Can you work these out from the model? Positions are in its coordinate system, mm. Face numbers are marked on the shaded views. Round coordinates to 2 decimals unless told otherwise and drop trailing zeros. Write each loop counter-clockwise with the first axis right and the second up, starting at its lowest first coordinate (ties: lowest second). Pieces come first, ordered by that corner, then holes. Notation, with made-up numbers: M 38.5,17.5 L 49.5,17.5 A27 ccw 49.5,48.5 Z; hole C 1.5,86.5 d1. An arc over 180 degrees is marked long. Answer in a Markdown table with one row per item. Add a question column.
(1) If we mould it in two halves opening along Z, with no side actions, what happens to the marked faces 1, 2 and 3? For each: released by +Z, released by -Z, zero draft, split by the parting line, or undercut.
(2) I'm going to push flat-ended pins straight in: pin 1 (4 mm diameter, centred on x = 23, y = 44.5, fed in from +Z); pin 2 (8 mm diameter, centred on y = 57.5, z = -13.5, fed in from +X); pin 3 (2.5 mm diameter, centred on x = 9.29, y = 58, fed in from -Z); pin 4 (4 mm diameter, centred on x = 23.5, y = 39, fed in from -Z). Where does each tip first touch, or does it pass through?
(3) Suppose I cut it at C-C, the plane x = 11.75. Write out the boundary of the cut face in (y, z), then the cut area to 3 significant figures.
(4) Suppose I cut it at A-A, the plane y = 64. Write out the boundary of the cut face in (x, z).
(5) Suppose I cut it at D-D, the plane z = -16.5. Write out the boundary of the cut face in (x, y), then the cut area to 3 significant figures.
(6) Suppose I cut it at B-B, the plane x = 8.5. Write out the boundary of the cut face in (y, z), then the cut area to 3 significant figures.
(7) If I drill on probe 1 along Y at (x, z) = (23, -9.7); probe 2 along Y at (x, z) = (8.5, -3.75); probe 3 along X at (y, z) = (63, -13.75), over which ranges is the centre line in solid material (lowest first)?
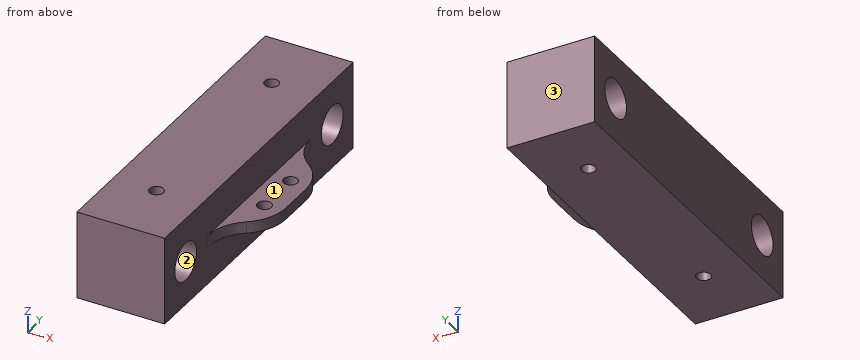
from build123d import *

# Parameters (mm, degrees)
SKETCH1_W           = 19
SKETCH1_H           = 19
BOSS_EXTRUDE1_DEPTH = 72
SKETCH2_R           = 4.15
CUT_EXTRUDE1_DEPTH  = 77.850504227
SKETCH3_R           = 1.5
CUT_EXTRUDE2_DEPTH  = 77.850504227
SKETCH4_W           = 2.5
SKETCH4_H           = 20
BOSS_EXTRUDE2_DEPTH = 8
FILLET1_R           = 10
FILLET2_R           = 10
SKETCH5_R           = 1.5
CUT_EXTRUDE3_DEPTH  = 10


with BuildPart() as part:
    # Sketch1 → Boss-Extrude1 (new body)
    with BuildSketch(Plane(origin=(0, 0, 0), x_dir=(1, 0, 0), z_dir=(0, 1, 0))):
        with Locations((9.5, 9.5)):
            Rectangle(SKETCH1_W, SKETCH1_H)
    extrude(amount=BOSS_EXTRUDE1_DEPTH)

    # Sketch2 → Cut-Extrude1 (cut, through all)
    with BuildSketch(Plane(origin=(19, 0, 0), x_dir=(0, 0, -1), z_dir=(1, 0, 0))):
        with Locations((9.5, 64)):
            Circle(SKETCH2_R)
        with Locations((9.5, 8)):
            Circle(SKETCH2_R)
    extrude(amount=-CUT_EXTRUDE1_DEPTH, mode=Mode.SUBTRACT)

    # Sketch3 → Cut-Extrude2 (cut, through all)
    with BuildSketch(Plane.XY):
        with Locations((9.290763855, 58)):
            Circle(SKETCH3_R)
        with Locations((9.290763855, 14)):
            Circle(SKETCH3_R)
    extrude(amount=-CUT_EXTRUDE2_DEPTH, mode=Mode.SUBTRACT)

    # Sketch4 → Boss-Extrude2 (add)
    with BuildSketch(Plane(origin=(19, 0, 0), x_dir=(0, 0, -1), z_dir=(1, 0, 0))):
        with Locations((9.5, 36)):
            Rectangle(SKETCH4_W, SKETCH4_H)
    extrude(amount=BOSS_EXTRUDE2_DEPTH)

    # Fillet1
    # the kernel refuses this fillet: 10 mm, written as the material it adds along each edge
    with BuildSketch(Plane(origin=(19, 46, -8.25), x_dir=(0, 1, 0), z_dir=(0, 0, -1)), Plane(origin=(19, 26, -10.75), x_dir=(0, -1, 0), z_dir=(0, 0, 1))) as fillet1_piece_1:
        with BuildLine():
            CenterArc((9.797958971, 10), FILLET1_R, 191.536959033, 78.463040967)
            Line((0, 8), (-0.195959179, 7.96))
            ThreePointArc((-0.195959179, 7.96), (-0.2, 4), (-0.2, 0))
            Line((-0.2, 0), (0, -0.2))
            Line((0, -0.2), (9.797958971, -0.2))
            Line((9.797958971, -0.2), (9.797958971, 0))
        make_face()
    extrude(amount=2.5)

    # Fillet2
    fillet2_edges = [part.edges().sort_by_distance(p)[0] for p in [
        (27, 46, -9.5),
        (27, 26, -9.5),
    ]]
    fillet(fillet2_edges, radius=FILLET2_R)

    # Sketch5 → Cut-Extrude3 (cut)
    with BuildSketch(Plane(origin=(0, 0, -10.75), x_dir=(-1, 0, 0), z_dir=(0, 0, -1))):
        with Locations((-23, 41)):
            Circle(SKETCH5_R)
        with Locations((-23, 31)):
            Circle(SKETCH5_R)
    extrude(amount=-CUT_EXTRUDE3_DEPTH, mode=Mode.SUBTRACT)


solid = part.part
Calculated:
| question | item | result |
|---|---|---|
| 1 | face 1 | released by +Z |
| 1 | face 2 | undercut |
| 1 | face 3 | zero draft |
| 2 | pin 1 | z = -8.25 |
| 2 | pin 2 | x = 19.07 |
| 2 | pin 3 | through |
| 2 | pin 4 | z = -10.75 |
| 3 | outline | M 0,-19 L 72,-19 L 72,0 L 0,0 Z; hole C 8,-9.5 d8.3; hole C 64,-9.5 d8.3 |
| 3 | area | 1,260 mm² |
| 4 | outline | M 0,-19 L 19,-19 L 19,-13.65 L 0,-13.65 Z; M 0,-5.35 L 19,-5.35 L 19,0 L 0,0 Z |
| 5 | outline | M 0,0 L 19,0 L 19,72 L 0,72 Z; hole C 9.29,14 d3; hole C 9.29,58 d3 |
| 5 | area | 1,350 mm² |
| 6 | outline | M 0,-19 L 12.73,-19 L 12.73,0 L 0,0 Z; M 15.27,-19 L 56.73,-19 L 56.73,0 L 15.27,0 Z; M 59.27,-19 L 72,-19 L 72,0 L 59.27,0 Z; hole C 8,-9.5 d8.3; hole C 64,-9.5 d8.3 |
| 6 | area | 1,160 mm² |
| 7 | probe 1 | 24.2 to 29.5, 32.5 to 39.5, 42.5 to 47.8 |
| 7 | probe 2 | 0 to 12.73, 15.27 to 56.73, 59.27 to 72 |
| 7 | probe 3 | 0 to 19 |
